```python
from build123d import *

# Parameters (mm, degrees)
ESQUISSE1_W                                        = 50
ESQUISSE1_H                                        = 12
BOSS_EXTRU_1_DEPTH                                 = 10
ESQUISSE3_W                                        = 12
ESQUISSE3_H                                        = 12
BOSS_EXTRU_2_DEPTH                                 = 2
ENL_V_MAT_EXTRU_3_DEPTH                            = 29.372521918
ENL_V_MAT_EXTRU_3_DEPTH_BACK                       = 29.372521918
ESQUISSE4_W                                        = 18
ESQUISSE4_H                                        = 3.498401272
CHAMBRAGE_POUR_VIS_T_TE_HEXAGONALE_M52_D           = 5.5
CHAMBRAGE_POUR_VIS_T_TE_HEXAGONALE_M52_CBORE_D     = 10
CHAMBRAGE_POUR_VIS_T_TE_HEXAGONALE_M52_CBORE_DEPTH = 5.4


with BuildPart() as part:
    # Esquisse1 → Boss.-Extru.1 (new body)
    with BuildSketch(Plane.XY):
        Rectangle(ESQUISSE1_W, ESQUISSE1_H)
    extrude(amount=BOSS_EXTRU_1_DEPTH)

    # Esquisse3 → Boss.-Extru.2 (add)
    with BuildSketch(Plane.XY.offset(10)):
        with Locations((-19, 0)):
            Rectangle(ESQUISSE3_W, ESQUISSE3_H)
    extrude(amount=BOSS_EXTRU_2_DEPTH)

    # Esquisse4 → Enlèv. mat.-Extru.3 (cut, two sides: drawn at the far end of the back side and taken through both)
    with BuildSketch(Plane(origin=(0, 0, 0), x_dir=(1, 0, 0), z_dir=(0, 1, 0)).offset(-ENL_V_MAT_EXTRU_3_DEPTH_BACK)):
        with Locations((0, 0.749200636)):
            Rectangle(ESQUISSE4_W, ESQUISSE4_H)
    extrude(amount=ENL_V_MAT_EXTRU_3_DEPTH + ENL_V_MAT_EXTRU_3_DEPTH_BACK, mode=Mode.SUBTRACT)

    # Chambrage pour vis à tête hexagonale M52 (through all)
    with Locations(Plane(origin=(0, 0, 0), x_dir=(-1, 0, 0), z_dir=(0, 0, -1))):
        with Locations((18, 0)):
            CounterBoreHole(CHAMBRAGE_POUR_VIS_T_TE_HEXAGONALE_M52_D / 2, CHAMBRAGE_POUR_VIS_T_TE_HEXAGONALE_M52_CBORE_D / 2, CHAMBRAGE_POUR_VIS_T_TE_HEXAGONALE_M52_CBORE_DEPTH)


solid = part.part
```
The model under review builds one solid part; all positions refer to its coordinate system, in mm. A direction names the side the tool comes from. Round coordinates to 2 decimals unless told otherwise and drop trailing zeros. Write each loop counter-clockwise with the first axis right and the second up, starting at its lowest first coordinate (ties: lowest second). Pieces come first, ordered by that corner, then holes. Notation, with made-up numbers: (78.25, -13.5) - (118.25, -13.5) arc R18 cw to (118.25, 11.5) - close; hole circle Ø8 at (-21, 25). An arc over 180 degrees is marked (long way). Use one line per item in the form item = value.
Q1. Insertion check: pin 1 Ø1.5 at (x, y) = (6.5, -1) entering from +Z. The pin has a flat end and moves straight along its axis. Give the tip position at first contact, or say it passes through.
Answer key:
pin_1 = 10
Q2. Consider section C-C (y = 0). State the section outline as (x, z) points.
Answer key:
outline = (-25, 0) - (-23, 0) - (-23, 5.4) - (-20.75, 5.4) - (-20.75, 12) - (-25, 12) - close; (-15.25, 5.4) - (-13, 5.4) - (-13, 0) - (-9, 0) - (-9, 1) - (9, 1) - (9, 0) - (25, 0) - (25, 10) - (-13, 10) - (-13, 12) - (-15.25, 12) - close
Q3. Consider section B-B (z = 9.5). State the section outline as (x, y) points.
Answer key:
outline = (-25, -6) - (25, -6) - (25, 6) - (-25, 6) - close; hole circle Ø5.5 at (-18, 0)
Q4. For line 1 (Y direction, x = -18, z = 3.8); line 2 (Y direction, x = -18, z = 7.5); line 3 (Z direction, x = -3, y = -5.5), list the stretches that pass through material, from the lowest coordinate up. Write a range as [from, to].
Answer key:
line_1 = [-6, -5], [5, 6]
line_2 = [-6, -2.75], [2.75, 6]
line_3 = [1, 10]
Q5. Consider section D-D (z = 4.25). State the section outline as (x, y) points, and give its area (3 significant figures).
Answer key:
outline = (-25, -6) - (25, -6) - (25, 6) - (-25, 6) - close; hole circle Ø10 at (-18, 0)
area = 521 mm2
Q6. Tool access review of faces 1 (the flat face through (-20.2, -2.2, 5.4)), 2 (the flat face through (0, 0, 1)), 3 (the flat face through (6, 0, 10)), 4 (the cylindrical face through (-20.747, 0.121, 8.746)): name each direction out of +Z, -Z, +X, -X, +Y, -Y from which nothing blocks a thin tool from reaching the whole face with its end or side.
Answer key:
face_1 = -Z
face_2 = -Z, +Y, -Y
face_3 = +Z, +X, +Y, -Y
face_4 = +Z, -Z
Q7. Consider section A-A (x = -18). State the section outline as (y, z) points, and give its area (3 significant figures).
Answer key:
outline = (-6, 0) - (-5, 0) - (-5, 5.4) - (-2.75, 5.4) - (-2.75, 12) - (-6, 12) - close; (2.75, 5.4) - (5, 5.4) - (5, 0) - (6, 0) - (6, 12) - (2.75, 12) - close
area = 53.7 mm2
Q8. Draft analysis for pull direction Y (two halves, no side actions). For faces 5 (the cylindrical face through (-13, 0, 3)), 6 (the flat face through (-13, 0, 11)), 7 (the flat face through (0, 6, 6)), state which applies: +Y half, -Y half, draft (parallel to the pull), parting line (faces both ways), or undercut.
Answer key:
face_5 = undercut
face_6 = draft
face_7 = +Y half
